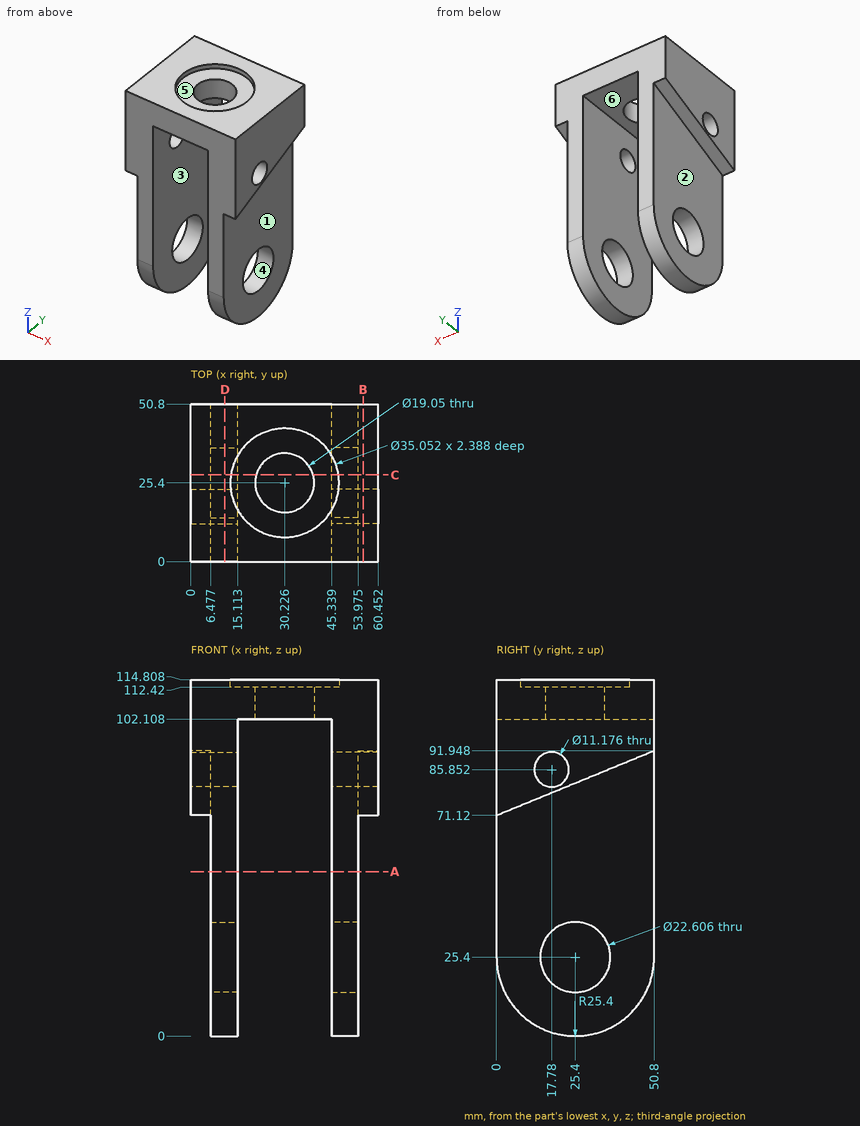
Geometry: see drawing. Coordinates: mm, zero at the bounding-box minimum. A direction names the side the tool comes from. Round coordinates to 2 decimals unless told otherwise and drop trailing zeros. Loops run counter-clockwise (first coordinate to the right, second up) from the corner with the lowest first, then second, coordinate; pieces in that order, holes last. Notation, with made-up numbers: (35.25, 25.5) - (70.25, 25.5) arc R17 cw to (70.25, 36.5) - close; hole circle Ø5 at (-39.5, -2). An arc over 180 degrees is marked (long way). One line per item, written item: value. Start each with the question number.
(1) Access query for the marked faces 4, 5 and 6. Directions: +Z, -Z, +X, -X, +Y, -Y. A direction counts if a zero-diameter tool reaches every point of the face in a straight line with its end or side. Return the directions, or none.
(2) Ray query, line 1 (X direction, y = 32, z = 75.5) (1 decimal); line 2 (Z direction, x = 35, y = 7); line 3 (Z direction, x = 9, y = 21.5). Return the intervals inside material, ascending. Write a range as [from, to].
(3) Section D-D, the plane x = 11. Return loops of the section in (y, z), plus the area to 3 significant figures.
(4) Section C-C, the plane y = 28. Return loops of the section in (x, z) (1 decimal).
(5) Section A-A, the plane z = 53. Return loops of the section in (x, y) (1 decimal).
(6) Section B-B, the plane x = 55.5. Return loops of the section in (y, z), plus the area to 3 significant figures.
(7) Draft query along X for the marked faces 1, 2 and 3. Return one class per face: +X half, -X half, draft (parallel to the pull), parting line (faces both ways), or undercut.
(8) Contact query for flat-ended pins moving along their axis: P1, Ø1, axis at y = 24.5, z = 49, coming from the +X side (3 decimals); P2, Ø13.5, axis at y = 25.4, z = 25.4, coming from the +X side; P3, Ø25, axis at x = 30.226, y = 25.4, coming from the -Z side; P4, Ø1, axis at x = 35.5, y = 11, coming from the +Z side. Output: stop coordinate, or through.
Results below:
1. face 4: +X, -X
1. face 5: +Z
1. face 6: -Z, +Y, -Y
2. line 1: [6.5, 15.1], [45.3, 54]
2. line 2: [102.11, 114.81]
2. line 3: [0.3, 14.79], [36.01, 81.68], [90.02, 114.81]
3. outline: (0, 25.4) arc R25.4 ccw to (50.8, 25.4) - (50.8, 114.81) - (0, 114.81) - close; hole circle Ø11.18 at (17.78, 85.85); hole circle Ø22.61 at (25.4, 25.4)
3. area: 5,060 mm^2
4. outline: (0, 82.6) - (6.5, 82.6) - (6.5, 36.4) - (15.1, 36.4) - (15.1, 102.1) - (21.1, 102.1) - (21.1, 112.4) - (12.9, 112.4) - (12.9, 114.8) - (0, 114.8) - close; (6.5, 0.1) - (15.1, 0.1) - (15.1, 14.4) - (6.5, 14.4) - close; (39.4, 102.1) - (45.3, 102.1) - (45.3, 36.4) - (54, 36.4) - (54, 82.6) - (60.5, 82.6) - (60.5, 114.8) - (47.6, 114.8) - (47.6, 112.4) - (39.4, 112.4) - close; (45.3, 0.1) - (54, 0.1) - (54, 14.4) - (45.3, 14.4) - close
5. outline: (6.5, 0) - (15.1, 0) - (15.1, 50.8) - (6.5, 50.8) - close; (45.3, 0) - (54, 0) - (54, 50.8) - (45.3, 50.8) - close
6. outline: (0, 71.12) - (50.8, 91.95) - (50.8, 114.81) - (0, 114.81) - close; hole circle Ø11.18 at (17.78, 85.85)
6. area: 1,590 mm^2
7. face 1: +X half
7. face 2: -X half
7. face 3: undercut
8. P1: x = 53.975
8. P2: through
8. P3: z = 102.11
8. P4: z = 112.42
